Geometry check sheet. Reference: the model listing, model coordinates, mm. Round coordinates to 2 decimals unless told otherwise and drop trailing zeros. Order: outer loops, then holes, each group sorted by start corner. A loop starts at its lowest first (then second) coordinate and runs counter-clockwise, first axis right, second up. Notation, with made-up numbers: (7.5, 89.5) - (18.5, 89.5) arc R16 ccw to (18.5, 104.5) - close; hole circle Ø6 at (-6, 64.25). An arc over 180 degrees is marked (long way). Return JSON: item names as keys, results as strings. Group by question number.
Q1. Material ranges on line 1 along X through (y, z) = (1.6, 0); line 2 along X through (y, z) = (27.5, -6.75); line 3 along Y through (x, z) = (63, 3.75), recorded low to high.
Q2. Sectioned sample at A-A, the plane x = -49.5. Record the cut outline in (y, z), then the cut area to 3 significant figures.
Q3. Sectioned sample at D-D, the plane y = 34.5. Record the cut outline in (x, z), then the cut area to 3 significant figures.
Q4. Sectioned sample at C-C, the plane x = 0. Record the cut outline in (y, z), then the cut area to 3 significant figures.
Q5. Gauge pin test, flat ends, axial feed: pin 1 Ø2.5 at (x, y) = (-46, 2.5) entering from -Z; pin 2 Ø1.5 at (x, y) = (-52, 2.5) entering from +Z; pin 3 Ø4 at (y, z) = (106.5, 3.5) entering from +X. Record the tip position at first contact, or that the pin passes through.
Q6. Sectioned sample at B-B, the plane z = 0. Record the cut outline in (x, y), then the cut area to 3 significant figures.
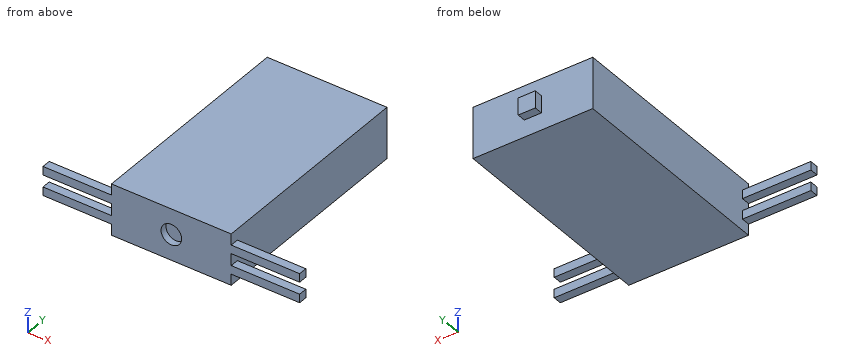
```python
from build123d import *

# Parameters (mm, degrees)
SKETCH2_W           = 70
SKETCH2_H           = 30
BOSS_EXTRUDE1_DEPTH = 127
SKETCH3_W           = 5
SKETCH3_H           = 5
BOSS_EXTRUDE2_DEPTH = 40
SKETCH4_W           = 5
SKETCH4_H           = 5
BOSS_EXTRUDE3_DEPTH = 40
SKETCH5_W           = 10
SKETCH5_H           = 10
BOSS_EXTRUDE4_DEPTH = 5
SKETCH6_R           = 6
CUT_EXTRUDE1_DEPTH  = 4


with BuildPart() as part:
    # Sketch2 → Boss-Extrude1 (new body)
    with BuildSketch(Plane(origin=(0, 0, 0), x_dir=(1, 0, 0), z_dir=(0, 1, 0))):
        Rectangle(SKETCH2_W, SKETCH2_H)
    extrude(amount=BOSS_EXTRUDE1_DEPTH)

    # Sketch3 → Boss-Extrude2 (add)
    with BuildSketch(Plane(origin=(35, 0, 0), x_dir=(0, 0, -1), z_dir=(1, 0, 0))):
        with Locations((-6, 2.5)):
            Rectangle(SKETCH3_W, SKETCH3_H)
        with Locations((6, 2.5)):
            Rectangle(SKETCH3_W, SKETCH3_H)
    extrude(amount=BOSS_EXTRUDE2_DEPTH)

    # Sketch4 → Boss-Extrude3 (add)
    with BuildSketch(Plane.ZY.offset(35)):
        with Locations((-6, 2.5)):
            Rectangle(SKETCH4_W, SKETCH4_H)
        with Locations((6, 2.5)):
            Rectangle(SKETCH4_W, SKETCH4_H)
    extrude(amount=BOSS_EXTRUDE3_DEPTH)

    # Sketch5 → Boss-Extrude4 (add)
    with BuildSketch(Plane(origin=(0, 127, 0), x_dir=(1, 0, 0), z_dir=(0, 1, 0))):
        Rectangle(SKETCH5_W, SKETCH5_H)
    extrude(amount=BOSS_EXTRUDE4_DEPTH)

    # Sketch6 → Cut-Extrude1 (cut)
    with BuildSketch(Plane(origin=(0, 0, 0), x_dir=(-1, 0, 0), z_dir=(0, -1, 0))):
        with Locations(Location((0, 0, 0), (0, 0, 90))):
            Circle(SKETCH6_R)
    extrude(amount=-CUT_EXTRUDE1_DEPTH, mode=Mode.SUBTRACT)


solid = part.part
```
Reply:
{
 "1": {"line 1": "-35 to -6, 6 to 35", "line 2": "-35 to 35", "line 3": "0 to 5"},
 "2": {"outline": "(0, -8.5) - (5, -8.5) - (5, -3.5) - (0, -3.5) - close; (0, 3.5) - (5, 3.5) - (5, 8.5) - (0, 8.5) - close", "area": "50.0 mm^2"},
 "3": {"outline": "(-35, -15) - (35, -15) - (35, 15) - (-35, 15) - close", "area": "2,100 mm^2"},
 "4": {"outline": "(0, -15) - (127, -15) - (127, -5) - (132, -5) - (132, 5) - (127, 5) - (127, 15) - (0, 15) - (0, 6) - (4, 6) - (4, -6) - (0, -6) - close", "area": "3,810 mm^2"},
 "5": {"pin 1": "z = -8.5", "pin 2": "z = 8.5", "pin 3": "x = 35"},
 "6": {"outline": "(-35, 0) - (-6, 0) - (-6, 4) - (6, 4) - (6, 0) - (35, 0) - (35, 127) - (5, 127) - (5, 132) - (-5, 132) - (-5, 127) - (-35, 127) - close", "area": "8,890 mm^2"}
}
